The listing builds one solid part. Answer for the finished solid, in the listing's coordinates (mm). Face numbers are marked on the shaded views. A direction names the side the tool comes from. Give positions to 0.01 mm unless a question says otherwise; leave off trailing zeros. Write each loop counter-clockwise with the first axis right and the second up, starting at its lowest first coordinate (ties: lowest second). Pieces come first, ordered by that corner, then holes. Notation, with made-up numbers: (53, 78.5) - (112, 78.5) arc R22 ccw to (112, 92.5) - close; hole circle Ø5 at (40.25, 52.25). An arc over 180 degrees is marked (long way). Answer as CSV lines item,"result". Start each with the question number.
(1) For the marked faces 1 and 2, determine the directions among +Z, -Z, +X, -X, +Y, -Y from which every point of the face is accessible in a straight line to the end or side of a thin tool.
(2) Find section C-C (x = 6.5). Write down the section's boundary in (y, z), then the cut area to 3 significant figures.
(3) Each of these flat-tipped pins is pushed along its axis until it touches: pin 1 Ø1.5 at (x, y) = (65.5, -2.5) entering from -Z; pin 2 Ø2 at (x, y) = (64, -1.5) entering from -Z; pin 3 Ø6 at (x, z) = (36.5, 4.5) entering from +Y. Where does it stop, or does it pass through?
(4) Find section A-A (y = 0). Write down the section's boundary in (x, z), then the cut area to 3 significant figures.
(5) Find section B-B (x = 28.5). Write down the section's boundary in (y, z), then the cut area to 3 significant figures.
(6) Straight lines are drawn through the part: probe 1 along X at (y, z) = (-3.5, -2); probe 2 along X at (y, z) = (2.75, 0); probe 3 along Y at (x, z) = (34, 0.25). For each, find the intervals that lie inside material, in ascending order.
from build123d import *

# Parameters (mm, degrees)
F0_W    = 14
F0_H    = 3.9
F2_SIZE = 0.5
F3_SIZE = 0.1
F4_SIZE = 0.3


# Not quite as in the source:
# - a fillet or chamfer that OpenCascade refuses, or shapes differently, is made with other operations: its cross-section is extruded or revolved along the edge and cut away or added


with BuildPart() as f1:
    # F0 (on Front) → F1 (revolve)
    with BuildSketch(Plane.XZ):
        Polygon((0, 1.5), (0, 0), (71, 0), (71, 3.9), (16, 3.9), (16, 6), (13, 6), (13, 3.9), (7.5, 3.9), (4.1531170718, 1.5), align=None)
        with Locations((78, 1.95)):
            Rectangle(F0_W, F0_H)
    revolve(axis=Axis((35.5, 0, 0), (1, 0, 0)))

    # F2
    f2_edges = [f1.edges().sort_by_distance(p)[0] for p in [
        (16, 0, -6),
    ]]
    chamfer(f2_edges, length=F2_SIZE)

    # F3
    f3_edges = [f1.edges().sort_by_distance(p)[0] for p in [
        (13, 0, -6),
    ]]
    chamfer(f3_edges, length=F3_SIZE)

    # F4
    f4_edges = [f1.edges().sort_by_distance(p)[0] for p in [
        (0, 0, -1.5),
    ]]
    chamfer(f4_edges, length=F4_SIZE)

    # F5: chamfer of 1 on 2 edges, made by hand

    # F5_s1 → F5_t2 (revolve, cut)
    with BuildSketch(Plane.XZ):
        Polygon((15.7071067812, 5.7928932188), (16, 5.0857864376), (16, 5.5), align=None)
    revolve(axis=Axis((16, 0, 0), (1, 0, 0)), mode=Mode.SUBTRACT)

    # F5_s3 → F5_t4 (revolve, cut)
    with BuildSketch(Plane.XZ):
        Polygon((84, 3.9), (85, 2.9), (85, 3.9), align=None)
    revolve(axis=Axis((85, 0, 0), (1, 0, 0)), mode=Mode.SUBTRACT)


solid = f1.part
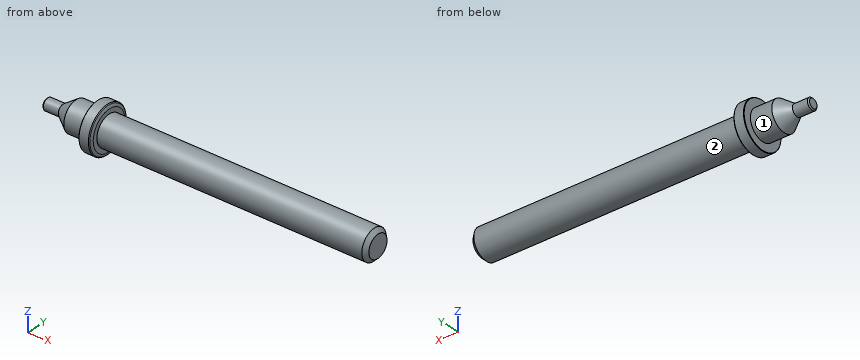
Result set:
1,face 1,"-X"
1,face 2,"+X"
2,outline,"circle Ø6.37 at (0, 0)"
2,area,"31.8 mm^2"
3,pin 1,"z = -3.49"
3,pin 2,"z = -3.87"
3,pin 3,"y = 3.6"
4,outline,"(0, -1.2) - (0.3, -1.5) - (4.15, -1.5) - (7.5, -3.9) - (13, -3.9) - (13, -5.9) - (13.1, -6) - (15.5, -6) - (15.71, -5.79) - (16, -5.09) - (16, -3.9) - (84, -3.9) - (85, -2.9) - (85, 2.9) - (84, 3.9) - (16, 3.9) - (16, 5.09) - (15.71, 5.79) - (15.5, 6) - (13.1, 6) - (13, 5.9) - (13, 3.9) - (7.5, 3.9) - (4.15, 1.5) - (0.3, 1.5) - (0, 1.2) - close"
4,area,"646 mm^2"
5,outline,"circle Ø7.8 at (0, 0)"
5,area,"47.8 mm^2"
6,probe 1,"13 to 16"
6,probe 2,"5.9 to 85"
6,probe 3,"-3.89 to 3.89"
